from build123d import *

# Parameters (mm, degrees)
F0_R      = 63.5
F1_DEPTH  = 6.35
F1_FACE_R = 63.5
F2_DEPTH  = 6.35
F3_R      = 6.35
F4_DEPTH  = 12.7
F3_R_2    = 25.4
F5_DEPTH  = 38.1
F6_R      = 12.7
F7_DEPTH  = 12.7
F8_R      = 6.35
F9_DEPTH  = 63.5


with BuildPart() as f1:
    # F0 (on Top) → F1 (new body)
    with BuildSketch(Plane.XY):
        Circle(F0_R)
    extrude(amount=F1_DEPTH)

    # F1_face (on face) → F2 (join)
    with BuildSketch(Plane(origin=(0, 0, 0), x_dir=(1, 0, 0), z_dir=(0, 0, -1))):
        Circle(F1_FACE_R)
    extrude(amount=F2_DEPTH)

    # F3 (on face) → F4 (cut)
    with BuildSketch(Plane.XY.offset(6.35)):
        with Locations((-44.45, 0)):
            Circle(F3_R)
        with Locations((0, 44.45)):
            Circle(F3_R)
        with Locations((44.45, 0)):
            Circle(F3_R)
        with Locations((0, -44.45)):
            Circle(F3_R)
    extrude(amount=-F4_DEPTH, mode=Mode.SUBTRACT)

    # F3 (on face) → F5 (join)
    with BuildSketch(Plane.XY.offset(6.35)):
        Circle(F3_R_2)
    extrude(amount=F5_DEPTH)

    # F6 (on face) → F7 (join)
    with BuildSketch(Plane.XY.offset(44.45)):
        Circle(F6_R)
    extrude(amount=F7_DEPTH)

    # F8 (on face) → F9 (cut)
    with BuildSketch(Plane.XY.offset(57.15)):
        Circle(F8_R)
    extrude(amount=-F9_DEPTH, mode=Mode.SUBTRACT)


solid = f1.part
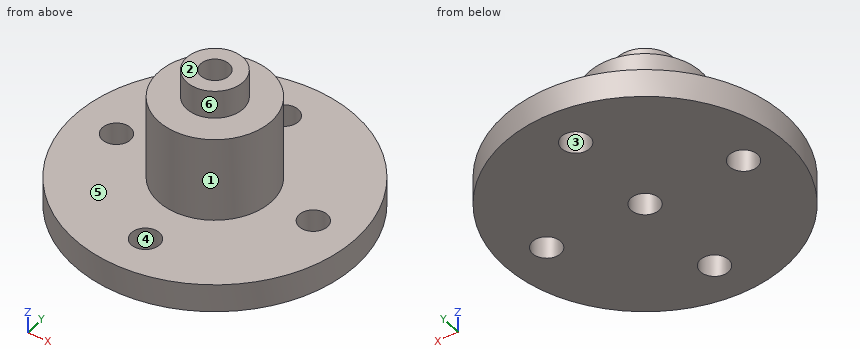
Model file for the job. Use its own axes, mm. Face numbers are marked on the shaded views. A direction names the side the tool comes from. Give positions to 0.01 mm unless a question says otherwise; leave off trailing zeros. Loops run counter-clockwise (first coordinate to the right, second up) from the corner with the lowest first, then second, coordinate; pieces in that order, holes last.
Item 1: Which spindle directions (+Z, -Z, +X, -X, +Y, -Y) get a long thin tool onto all of the face, cutting with end or side? Do the marked faces 1 and 2. Say none if no direction does.
Check values:
face 1: +Z
face 2: +Z, +X, -X, +Y, -Y
Item 2: Slice it at D-D (y = 48.5). Write the cut outline in (x, z).
Check values:
outline: (-40.99, -6.35) - (-4.89, -6.35) - (-4.89, 6.35) - (-40.99, 6.35) - close; (4.89, -6.35) - (40.99, -6.35) - (40.99, 6.35) - (4.89, 6.35) - close
Item 3: Slice it at A-A (y = 0). Write the cut outline in (x, z), plus the area to 3 significant figures.
Check values:
outline: (-63.5, -6.35) - (-50.8, -6.35) - (-50.8, 6.35) - (-63.5, 6.35) - close; (-38.1, -6.35) - (-6.35, -6.35) - (-6.35, 57.15) - (-12.7, 57.15) - (-12.7, 44.45) - (-25.4, 44.45) - (-25.4, 6.35) - (-38.1, 6.35) - close; (6.35, -6.35) - (38.1, -6.35) - (38.1, 6.35) - (25.4, 6.35) - (25.4, 44.45) - (12.7, 44.45) - (12.7, 57.15) - (6.35, 57.15) - close; (50.8, -6.35) - (63.5, -6.35) - (63.5, 6.35) - (50.8, 6.35) - close
area: 2,740 mm2
Item 4: Drop flat-ended pins along their axis: P1, Ø12, axis at x = -18, z = 24, coming from the -Y side; P2, Ø1, axis at y = 1, z = 41, coming from the -X side; P3, Ø4, axis at y = 25.5, z = 13, coming from the -X side. Give the stop position or say it passes through.
Check values:
P1: stops at y = -22.39
P2: stops at x = -25.4
P3: stops at x = -9.64
Item 5: Slice it at C-C (z = 1.5). Write the cut outline in (x, y), plus the area to 3 significant figures.
Check values:
outline: circle Ø127 at (0, 0); hole circle Ø12.7 at (-44.45, 0); hole circle Ø12.7 at (0, -44.45); hole circle Ø12.7 at (0, 0); hole circle Ø12.7 at (0, 44.45); hole circle Ø12.7 at (44.45, 0)
area: 12,000 mm2
Item 6: Mould opens along X. For the marked faces 3, 4, 5 and 6 say: +X half, -X half, draft (parallel to the pull), parting line (faces both ways), or undercut.
Check values:
face 3: undercut
face 4: undercut
face 5: draft
face 6: parting line
Item 7: Drill centre lines: line 1 along Y through (x, z) = (0, -1); line 2 along Y through (x, z) = (0, 7); line 3 along Z through (x, y) = (-22, 28). Where is each one in solid material? Low to high.
Check values:
line 1: y = -63.5 to -50.8, -38.1 to -6.35, 6.35 to 38.1, 50.8 to 63.5
line 2: y = -25.4 to -6.35, 6.35 to 25.4
line 3: z = -6.35 to 6.35
